Input: part model. Units: mm. Frame: model coordinates. A direction names the side the tool comes from. Round coordinates to 2 decimals unless told otherwise and drop trailing zeros. Loops run counter-clockwise (first coordinate to the right, second up) from the corner with the lowest first, then second, coordinate; pieces in that order, holes last. Notation, with made-up numbers: M 34,32.5 L 69,32.5 A35 cw 69,67.5 Z; hole C 13,15 d4. An arc over 180 degrees is marked long. Put each result on its own line as item: value. Start each with the question number.
1) Section B-B on z = 12.8. State how many separate pieces and enclosed holes the cut face has, plus the area to 3 significant figures.
2) Draft query along Y for faces 6 (the face through (-32.69, -7.124, 4.715)), 7 (the face through (-3, -16.639, 14)), 8 (the face through (0.008, -15.869, 1.065)). Return one class per face: +Y half, -Y half, draft (parallel to the pull), parting line (faces both ways), or undercut.
3) Reachability of faces 1 (the face through (-32.706, -17.738, 4.715)), 2 (the face through (-9, -13.939, 14)), 3 (the face through (-3.3, -13.4, 2.1)), 4 (the face through (-35.82, -13.31, 1.06)), 5 (the face through (-35, -16.439, 1)) from +Z, -Z, +X, -X, +Y, -Y: full face, straight path, thin tool, end or side. Return the list, or none.
4) Section D-D on z = 3. Output: boundary loops of the cut face in (x, y).
5) Line query: probe 1 along X at (y, z) = (-17.15, 12.8); probe 2 along Y at (x, z) = (-9, 14.25); probe 3 along Y at (x, z) = (-2.5, 2). Output: solid intervals per line, ascending.
6) Section A-A on y = -12. Output: boundary loops of the cut face in (x, z), plus the area to 3 significant figures.
7) Pin query (flat end, axial travel): pin 1 (2 mm diameter, centred on y = -15, z = 6, fed in from +X); pin 2 (3 mm diameter, centred on y = -10, z = 14.5, fed in from -X); pin 3 (1 mm diameter, centred on x = -34.5, z = 0.5, fed in from -Y). Return the tip coordinate at first contact, or that it passes through.
8) Section C-C on x = -26. Output: boundary loops of the cut face in (y, z), plus the area to 3 significant figures.
Autodesk Inventor part; units mm, degrees
ref_plane "YZ Plane" through (0, 0, 0) normal (1, 0, 0) x (0, 1, 0)
ref_plane "XZ Plane" through (0, 0, 0) normal (0, 1, 0) x (-1, 0, 0)
ref_plane "XY Plane" through (0, 0, 0) normal (0, 0, 1) x (1, 0, 0)
sketch "スケッチ1" plane through (0, 0, 0) normal (0, 0, 1) x (1, 0, 0)
  line L0 (-39.4908, -6.839) -> (0.6092, -6.839)
  line L1 (0.6092, -6.839) -> (0.6092, -18.039)
  line L2 (0.6092, -18.039) -> (-39.4908, -18.039)
  line L3 (-39.4908, -18.039) -> (-39.4908, -6.839)
  point P0 (0, 0)
  dimension "d0" = 40.1
  dimension "d1" = 11.2
extrude "押し出し1" add sketch "スケッチ1" along normal blind 16.3
sketch "スケッチ2" plane through (0.6092, -18.039, 0) normal (1, 0, 0) x (0, 0, -1)
  line L0 (-16.3, 11.2) -> (-16.3, 0)
  line L1 (0, 0) -> (-16.3, 0)
  line L2 (0, 11.2) -> (0, 0)
  line L3 (0, 11.2) -> (-16.3, 11.2)
  line L4 (-16.3, 0) -> (-9.3, 0)
  line L5 (-9.3, 0) -> (-9.3, 1.4)
  line L6 (-9.3, 1.4) -> (-16.3, 1.4)
  line L7 (-16.3, 1.4) -> (-16.3, 0)
  line L8 (-16.3, 11.2) -> (-9.3, 11.2)
  line L9 (-9.3, 11.2) -> (-9.3, 9.8)
  line L10 (-9.3, 9.8) -> (-16.3, 9.8)
  line L11 (-16.3, 9.8) -> (-16.3, 11.2)
  line L12 (0, 1.6) -> (-2.1, 1.6)
  line L13 (-2.1, 1.6) -> (-2.1, 9.6)
  line L14 (-2.1, 9.6) -> (0, 9.6)
  line L15 (0, 9.6) -> (0, 1.6)
  point P0 (0, 18.039)
  dimension "d4" = 8
  dimension "d5" = 2.1
  dimension "d6" = 7
  dimension "d7" = 7
  dimension "d8" = 8.4
extrude "押し出し2" cut sketch "スケッチ2" against normal blind 6.5 contours L10 L9 L3 L2 L14 L13 L12 L1 L5 L6 L0
sketch "スケッチ3" plane through (-39.4908, -18.039, 0) normal (-1, 0, 0) x (0, 0, 1)
  line L0 (16.3, 0) -> (16.3, 11.2)
  line L1 (0, 11.2) -> (16.3, 11.2)
  line L2 (0, 0) -> (0, 11.2)
  line L3 (0, 0) -> (16.3, 0)
  line L4 (16.3, 11.2) -> (9.3, 11.2)
  line L5 (9.3, 11.2) -> (9.3, 9.8)
  line L6 (9.3, 9.8) -> (16.3, 9.8)
  line L7 (16.3, 9.8) -> (16.3, 11.2)
  line L8 (16.3, 0) -> (9.3, 0)
  line L9 (9.3, 0) -> (9.3, 1.4)
  line L10 (9.3, 1.4) -> (16.3, 1.4)
  line L11 (16.3, 1.4) -> (16.3, 0)
  line L12 (0, 9.6) -> (2.1, 9.6)
  line L13 (2.1, 9.6) -> (2.1, 1.6)
  line L14 (2.1, 1.6) -> (0, 1.6)
  line L15 (0, 1.6) -> (0, 9.6)
  line L16 (2.1, 5.6) -> (16.3, 5.6)
  point P0 (0, 18.039)
  dimension "d12" = 7
  dimension "d13" = 7
  dimension "d14" = 8
  dimension "d15" = 2.1
  dimension "d16" = 8.4
  dimension "d17" = 4.2
extrude "押し出し3" cut sketch "スケッチ3" against normal blind 6.5 contours L10 L9 L3 L2 L14 L13 L16 L0 | L16 L13 L12 L2 L1 L5 L6 L0
sketch "スケッチ4" plane through (0, 0, 0) normal (0, 0, -1) x (-1, 0, 0)
  line L0 (5.8908, -18.039) -> (32.9908, -18.039)
  line L1 (39.4908, -8.439) -> (32.9908, -8.439)
  line L2 (36.4908, -12.439) -> (2.3908, -12.439)
  line L3 (19.4408, -12.439) -> (19.4408, -18.039)
  point P0 (0, 0)
  dimension "d20" = 34.1
  dimension "d21" = 5.6
hole "穴1" at (-36.4908, -12.439, 0) at (-2.3908, -12.439, 0) direction (0, 0, 1) diameter 2.2 end through all
sketch "スケッチ5" plane through (-39.4908, -18.039, 16.3) normal (0, -1, 0) x (1, 0, 0)
  line L0 (33.6, -16.3) -> (6.5, -16.3)
  line L1 (40.1, -7) -> (40.1, 0)
  line L2 (40.1, 0) -> (0, 0)
  line L3 (3, -3.5) -> (37.1, -3.5)
  line L4 (20.05, -3.5) -> (20.05, 0)
  point P0 (39.4908, -16.3)
  dimension "d29" = 34.1
  dimension "d30" = 12.8
hole "穴2" at (-36.4908, -18.039, 12.8) at (-2.3908, -18.039, 12.8) direction (0, 1, 0) diameter 2.2 end through all
fillet "フィレット1" radius 2 12 edges at (0.6092, -17.339, 16.3) (0.6092, -17.339, 9.3) (0.6092, -7.539, 16.3) (0.6092, -7.539, 9.3) (-39.4908, -7.539, 16.3) (-39.4908, -17.339, 16.3) (-39.4908, -17.339, 9.3) (-39.4908, -7.539, 9.3) (0.6092, -16.439, 1.05) (0.6092, -8.439, 1.05) (-39.4908, -16.439, 1.05) (-39.4908, -8.439, 1.05)
fillet "フィレット2" radius 1 4 edges at (-32.9908, -18.039, 4.65) (-5.8908, -18.039, 4.65) (-5.8908, -6.839, 4.65) (-32.9908, -6.839, 4.65)
sketch "スケッチ6" plane through (0, 0, 16.3) normal (0, 0, 1) x (1, 0, 0)
  line L0 (-29.4408, -9.939) -> (-21.4408, -9.939)
  line L1 (-21.4408, -9.939) -> (-21.4408, -14.939)
  line L2 (-21.4408, -14.939) -> (-29.4408, -14.939)
  line L3 (-9.4408, -9.939) -> (-17.4408, -9.939)
  line L4 (-17.4408, -9.939) -> (-17.4408, -14.939)
  line L5 (-17.4408, -14.939) -> (-9.4408, -14.939)
  line L6 (-29.4408, -9.939) -> (-30.4408, -9.939)
  line L7 (-30.4408, -9.939) -> (-30.4408, -10.939)
  line L8 (-30.4408, -10.939) -> (-29.4408, -10.939)
  line L9 (-29.4408, -12.439) -> (-30.4408, -12.439)
  line L10 (-30.4408, -12.439) -> (-30.4408, -13.439)
  line L11 (-30.4408, -13.439) -> (-29.4408, -13.439)
  line L12 (-9.4408, -14.939) -> (-8.4408, -14.939)
  line L13 (-8.4408, -14.939) -> (-8.4408, -13.939)
  line L14 (-8.4408, -13.939) -> (-9.4408, -13.939)
  line L15 (-9.4408, -12.439) -> (-8.4408, -12.439)
  line L16 (-8.4408, -12.439) -> (-8.4408, -11.439)
  line L17 (-8.4408, -11.439) -> (-9.4408, -11.439)
  line L18 (-29.4408, -14.939) -> (-29.4408, -13.439)
  line L19 (-29.4408, -12.439) -> (-29.4408, -10.939)
  line L20 (-9.4408, -13.939) -> (-9.4408, -12.439)
  line L21 (-9.4408, -11.439) -> (-9.4408, -9.939)
  point P0 (0, 0)
  dimension "d41" = 5
  dimension "d43" = 1
  dimension "d46" = 1
  dimension "d47" = 1
  dimension "d50" = 1
extrude "押し出し4" cut sketch "スケッチ6" against normal blind 5
properties part number "TB-22PP" material "ABS Plastic"
Geometry results:
1. separate pieces: 5
1. enclosed holes: 2
1. area: 244 mm²
2. face 6: +Y half
2. face 7: undercut
2. face 8: -Y half
3. face 1: -Z, -X, -Y
3. face 2: +Z
3. face 3: +Z, +X, +Y, -Y
3. face 4: +Z, -Z
3. face 5: +Z, -Z, -X, -Y
4. outline: M -32.99,-17.04 A1 ccw -31.99,-18.04 L -6.89,-18.04 A1 ccw -5.89,-17.04 L -5.89,-7.84 A1 ccw -6.89,-6.84 L -31.99,-6.84 A1 ccw -32.99,-7.84 Z
5. probe 1: x = -39.49 to -37.59, -35.39 to -3.49, -1.29 to 0.61
5. probe 2: y = -18.04 to -14.94, -13.94 to -12.44, -11.44 to -6.84
5. probe 3: y = -16.44 to -13.53, -11.34 to -8.44
6. outline: M -39.49,0 L -37.5,0 L -37.5,2.1 L -39.49,2.1 Z; M -35.48,0 L -3.4,0 L -3.4,2.1 L -5.89,2.1 L -5.89,16.3 L -8.44,16.3 L -8.44,11.3 L -17.44,11.3 L -17.44,16.3 L -21.44,16.3 L -21.44,11.3 L -29.44,11.3 L -29.44,16.3 L -32.99,16.3 L -32.99,2.1 L -35.48,2.1 Z; M -1.38,0 L 0.61,0 L 0.61,2.1 L -1.38,2.1 Z
6. area: 376 mm²
7. pin 1: stops at x = -5.89
7. pin 2: stops at x = -32.99
7. pin 3: stops at y = -16.44
8. outline: M -18.04,0 L -6.84,0 L -6.84,16.3 L -9.94,16.3 L -9.94,11.3 L -14.94,11.3 L -14.94,16.3 L -18.04,16.3 Z
8. area: 158 mm²
